Geometry: final body of the model. Coordinates: model frame, mm. A direction names the side the tool comes from. Round coordinates to 2 decimals unless told otherwise and drop trailing zeros. Loops run counter-clockwise (first coordinate to the right, second up) from the corner with the lowest first, then second, coordinate; pieces in that order, holes last. Notation, with made-up numbers: (43, 68.5) - (56, 68.5) arc R31 ccw to (56, 94.5) - close; hole circle Ø4 at (0.5, 61.25). An arc over 180 degrees is marked (long way). Return JSON: item names as keys, results as strings. Group by question number.
1. Material intervals for probe 1 along X at (y, z) = (-7, -0.7); probe 2 along Z at (x, y) = (-14, -26); probe 3 along Z at (x, y) = (-8, -14.5), sorted ascending.
2. Section D-D on x = -14.75. Return loops of the section in (y, z), and give its area (3 significant figures).
3. Section C-C on y = -33. Return loops of the section in (x, z), and give its area (3 significant figures).
4. First-contact query: pin 1 Ø2.5 at (x, y) = (-14.92, -7) entering from +Z; pin 2 Ø3 at (x, y) = (5.5, -30) entering from +Z. Flat tips, straight axial feed; report the tip coordinate or a pass-through.
5. Draft query along Z for faces 6 (the face through (-7, -22, 2.5)), 7 (the face through (-18.918, -22, -1)), 8 (the face through (-1, -22, 7.5)). Return one class per face: +Z half, -Z half, draft (parallel to the pull), parting line (faces both ways), or undercut.
6. Section B-B on x = 4.5. Return loops of the section in (y, z).
7. Set-up query: faces 1 (the face through (-12, -22, 0)), 2 (the face through (-8.918, -22, 3)), 3 (the face through (-3, -45, 1)), 4 (the face through (4, -22, 2.5)), 5 (the face through (-3, 0, 1)). Return all of +Z, -Z, +X, -X, +Y, -Y with unobstructed straight access to the full face (end or side cutting, diameter ignored); none if empty.
8. Section A-A on y = -7. Return loops of the section in (x, z).
from build123d import *

# Parameters (mm, degrees)
F1_DEPTH = 45
F2_W     = 45
F2_H     = 3
F3_DEPTH = 10
F5_D     = 3.3


with BuildPart() as f1:
    # F0 (on Front) → F1 (new body)
    with BuildSketch(Plane.XZ):
        Polygon((-4.964183461, 2.5), (-4.964183461, 0), (2.535816539, 0), (2.535816539, 2.5), (6.4899705969, 2.5), (6.4899705969, 4), (2.535816539, 7.5), (-4.964183461, 7.5), (-8.9183375189, 4), (-8.9183375189, 2.5), align=None)
        Polygon((2.535816539, 0), (-4.964183461, 0), (-8.9183375189, 0), (-8.9183375189, -3), (6.4899705969, -3), (6.4899705969, 0), align=None)
    extrude(amount=F1_DEPTH)

    # F2 (on face) → F3 (join)
    with BuildSketch(Plane(origin=(-8.9183375189, 0, 0), x_dir=(0, -1, 0), z_dir=(-1, 0, 0))):
        with Locations((22.5, -1.5)):
            Rectangle(F2_W, F2_H)
    extrude(amount=F3_DEPTH)

    # F5 (through all)
    with Locations(Plane(origin=(0, 0, -3), x_dir=(1, 0, 0), z_dir=(0, 0, -1))):
        with Locations((-14.9183375189, 38), (-14.9183375189, 7)):
            Hole(F5_D / 2)


solid = f1.part
Taken from the geometry:
{
 "1": {"probe 1": "-18.92 to -16.57, -13.27 to 6.49", "probe 2": "-3 to 0", "probe 3": "-3 to 0, 2.5 to 4.81"},
 "2": {"outline": "(-45, -3) - (-39.64, -3) - (-39.64, 0) - (-45, 0) - close; (-36.36, -3) - (-8.64, -3) - (-8.64, 0) - (-36.36, 0) - close; (-5.36, -3) - (0, -3) - (0, 0) - (-5.36, 0) - close", "area": "115 mm2"},
 "3": {"outline": "(-18.92, -3) - (6.49, -3) - (6.49, 0) - (2.54, 0) - (2.54, 2.5) - (6.49, 2.5) - (6.49, 4) - (2.54, 7.5) - (-4.96, 7.5) - (-8.92, 4) - (-8.92, 2.5) - (-4.96, 2.5) - (-4.96, 0) - (-18.92, 0) - close", "area": "158 mm2"},
 "4": {"pin 1": "through", "pin 2": "z = 6.2"},
 "5": {"face 6": "undercut", "face 7": "draft", "face 8": "+Z half"},
 "6": {"outline": "(-45, -3) - (0, -3) - (0, 0) - (-45, 0) - close; (-45, 2.5) - (0, 2.5) - (0, 5.76) - (-45, 5.76) - close"},
 "7": {"face 1": "-X, +Y, -Y", "face 2": "+Z, -X, +Y, -Y", "face 3": "+Z, -Z, +X, -X, -Y", "face 4": "+X, +Y, -Y", "face 5": "+Z, -Z, +X, -X, +Y"},
 "8": {"outline": "(-18.92, -3) - (-16.57, -3) - (-16.57, 0) - (-18.92, 0) - close; (-13.27, -3) - (6.49, -3) - (6.49, 0) - (2.54, 0) - (2.54, 2.5) - (6.49, 2.5) - (6.49, 4) - (2.54, 7.5) - (-4.96, 7.5) - (-8.92, 4) - (-8.92, 2.5) - (-4.96, 2.5) - (-4.96, 0) - (-13.27, 0) - close"}
}
